Could you check a few things on this model? Use its own coordinates, in mm. Face numbers are marked on the shaded views. A direction names the side the tool comes from. Coordinates: 2 decimals unless noted, no trailing zeros. Write each loop counter-clockwise with the first axis right and the second up, starting at its lowest first coordinate (ties: lowest second). Pieces come first, ordered by that corner, then holes. Notation, with made-up numbers: M 29,-22.75 L 86,-22.75 A25 ccw 86,8.25 Z; hole C 45.25,11 d3. An arc over 180 degrees is marked long. Answer as CSV lines item,"result". Start each with the question number.
Item 1: If I drill on line 1 along Y through (x, z) = (-1.5, -5.25); line 2 along Z through (x, y) = (-51.5, -6); line 3 along Z through (x, y) = (-50, 1), over which ranges is the centre line in solid material (lowest first)? Write a range as [from, to].
Item 2: Suppose I cut it at C-C, the plane x = -60.5. Write out the boundary of the cut face in (y, z).
Item 3: Suppose I cut it at D-D, the plane y = -3. Write out the boundary of the cut face in (x, z) (1 decimal), and give its area (3 significant figures).
Item 4: Suppose I cut it at B-B, the plane z = -2.25. Write out the boundary of the cut face in (x, y).
Item 5: On a 3-axis mill with a long thin cutter (end or side, diameter ignored), from which of +Z, -Z, +X, -X, +Y, -Y can I reach the whole of each face in a straight line? I mean the marked faces 1 and 2. Say none if no direction works.
Item 6: I'm going to push flat-ended pins straight in: P1, Ø6, axis at x = 42.5, z = -16.5, coming from the -Y side; P2, Ø4, axis at x = 8.5, y = -4.5, coming from the -Z side. Where does each tip first touch, or does it pass through?
Item 7: Suppose I cut it at A-A, the plane y = 4.75. Write out the boundary of the cut face in (x, z) (1 decimal), and give its area (3 significant figures).
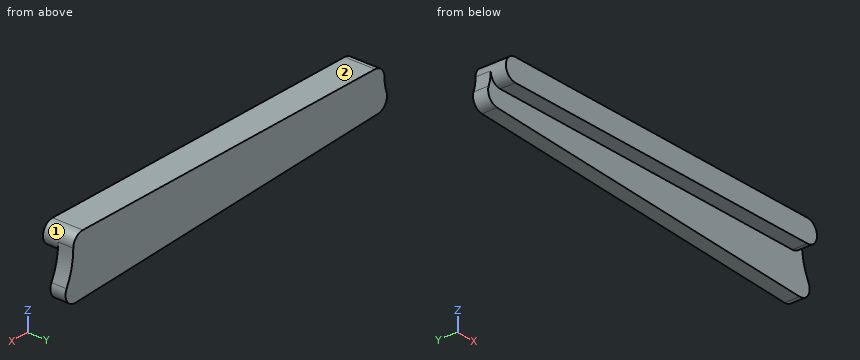
```python
from build123d import *

# Parameters (mm, degrees)
BOSS_EXTRUDE1_DEPTH = 6.499999954
BOSS_EXTRUDE2_DEPTH = 6.5


with BuildPart() as part:
    # Sketch1 → Boss-Extrude1 (new body, symmetric)
    with BuildSketch(Plane(origin=(0, 0, 0), x_dir=(1, 0, 0), z_dir=(0, 1, 0))):
        with BuildLine():
            Line((-73.025, 4.7625), (73.025, 4.7625))
            ThreePointArc((73.025, 4.7625), (77.7875, 0), (73.025, -4.7625))
            Line((73.025, -4.7625), (-73.025, -4.7625))
            ThreePointArc((-73.025, -4.7625), (-77.7875, 0), (-73.025, 4.7625))
        make_face()
    extrude(amount=BOSS_EXTRUDE1_DEPTH, both=True)

    # Sketch3 → Boss-Extrude2 (add)
    with BuildSketch(Plane(origin=(0, 0, 0), x_dir=(1, 0, 0), z_dir=(0, 1, 0))):
        with BuildLine():
            Line((76.658892628, 20.587985299), (-74.559016538, 12.30586185))
            ThreePointArc((-74.559016538, 12.30586185), (-78.253429498, 10.203877505), (-78.797570633, 5.988318736))
            ThreePointArc((-78.797570633, 5.988318736), (-78.041788633, 3.036453687), (-77.7875, 0))
            ThreePointArc((-77.7875, 0), (-76.392596045, 3.367596045), (-73.025, 4.7625))
            Line((-73.025, 4.7625), (73.025, 4.7625))
            ThreePointArc((73.025, 4.7625), (76.392596045, 3.367596045), (77.7875, 0))
            ThreePointArc((77.7875, 0), (78.637537914, 7.014737168), (81.13844531, 13.623410575))
            ThreePointArc((81.13844531, 13.623410575), (80.924845702, 18.408916837), (76.658892628, 20.587985299))
        make_face()
    extrude(amount=BOSS_EXTRUDE2_DEPTH)


solid = part.part
```
Ans:
1,line 1,"y = [0, 6.5]"
1,line 2,"z = [-4.76, 4.76]"
1,line 3,"z = [-13.65, 4.76]"
2,outline,"M -6.5,-4.76 L 0,-4.76 L 0,-13.08 L 6.5,-13.08 L 6.5,4.76 L -6.5,4.76 Z"
3,outline,"M -73,-4.8 L 73,-4.8 A4.8 ccw 73,4.8 L -73,4.8 A4.8 ccw Z"
3,area,"1,460 mm^2"
4,outline,"M -77.93,0 L -77.22,0 L -77.22,-6.5 L 77.22,-6.5 L 77.22,0 L 77.87,0 L 77.87,6.5 L -77.93,6.5 Z"
5,face 1,"+X, -Y"
5,face 2,"+Z, +X, -X, +Y, -Y"
6,P1,"stops at y = 0"
6,P2,"stops at z = -4.76"
7,outline,"M -78.8,-6 A4.8 ccw -74.6,-12.3 L 76.7,-20.6 A4.8 ccw 81.1,-13.6 A29.4 cw 77.8,0 A4.8 ccw 73,4.8 L -73,4.8 A4.8 ccw -77.8,0 A18.3 cw Z"
7,area,"3,320 mm^2"
